Design review of the part built by this model. Coordinates are the model's own, in mm. Give positions to 0.01 mm unless a question says otherwise; leave off trailing zeros. Order: outer loops, then holes, each group sorted by start corner. A loop starts at its lowest first (then second) coordinate and runs counter-clockwise, first axis right, second up. Notation, with made-up numbers: (80.25, 29) -> (138.25, 29) arc R7 cw to (138.25, 42) -> close; hole circle Ø6 at (46.5, 56.5). An arc over 180 degrees is marked (long way). Return JSON: item names as keys, results as strings.
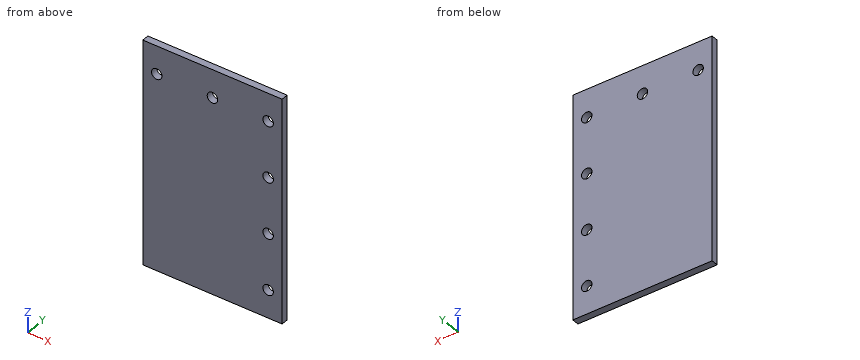
```python
from build123d import *

# Parameters (mm, degrees)
SKETCH1_W           = 63.5
SKETCH1_H           = 101.6
BOSS_EXTRUDE1_DEPTH = 3.175
SKETCH2_R           = 2.38125
CUT_EXTRUDE1_DEPTH  = 3.175


with BuildPart() as part:
    # Sketch1 → Boss-Extrude1 (new body)
    with BuildSketch(Plane(origin=(0, 0, 0), x_dir=(1, 0, 0), z_dir=(0, 1, 0))):
        Rectangle(SKETCH1_W, SKETCH1_H)
    extrude(amount=BOSS_EXTRUDE1_DEPTH)

    # Sketch2 → Cut-Extrude1 (cut)
    with BuildSketch(Plane(origin=(0, 3.175, 0), x_dir=(1, 0, 0), z_dir=(0, 1, 0))):
        with Locations(Location((25.4, -38.1, 0), (0, 0, 270))):
            Circle(SKETCH2_R)
        with Locations(Location((25.4, -12.7, 0), (0, 0, 270))):
            Circle(SKETCH2_R)
        with Locations(Location((25.4, 12.7, 0), (0, 0, 270))):
            Circle(SKETCH2_R)
        with Locations(Location((25.4, 38.1, 0), (0, 0, 270))):
            Circle(SKETCH2_R)
        with Locations(Location((0, -38.1, 0), (0, 0, 270))):
            Circle(SKETCH2_R)
        with Locations(Location((-25.4, -38.1, 0), (0, 0, 270))):
            Circle(SKETCH2_R)
        with Locations((-50.8, -38.1)):
            Circle(SKETCH2_R)
    extrude(amount=-CUT_EXTRUDE1_DEPTH, mode=Mode.SUBTRACT)


solid = part.part
```
Item 1: For pin 1 (3 mm diameter, centred on x = 25.4, z = 38.1, fed in from +Y), flat-tipped, find the tip position at first contact; note if it passes through.
Result set:
{"pin 1": "passes through"}
Item 2: Add section D-D (z = 12.7). Give the boundary of the cut face in (x, y) (3 decimals), plus the area to 3 significant figures.
Result set:
{"outline": "(-31.75, 0) -> (23.019, 0) -> (23.019, 3.175) -> (-31.75, 3.175) -> close; (27.781, 0) -> (31.75, 0) -> (31.75, 3.175) -> (27.781, 3.175) -> close", "area": "186 mm^2"}
Item 3: Add section A-A (x = 25.4). Give the boundary of the cut face in (y, z) (3 decimals), plus the area to 3 significant figures.
Result set:
{"outline": "(0, -50.8) -> (3.175, -50.8) -> (3.175, -40.481) -> (0, -40.481) -> close; (0, -35.719) -> (3.175, -35.719) -> (3.175, -15.081) -> (0, -15.081) -> close; (0, -10.319) -> (3.175, -10.319) -> (3.175, 10.319) -> (0, 10.319) -> close; (0, 15.081) -> (3.175, 15.081) -> (3.175, 35.719) -> (0, 35.719) -> close; (0, 40.481) -> (3.175, 40.481) -> (3.175, 50.8) -> (0, 50.8) -> close", "area": "262 mm^2"}
Item 4: Add section C-C (x = 0). Give the boundary of the cut face in (y, z) (3 decimals).
Result set:
{"outline": "(0, -50.8) -> (3.175, -50.8) -> (3.175, 35.719) -> (0, 35.719) -> close; (0, 40.481) -> (3.175, 40.481) -> (3.175, 50.8) -> (0, 50.8) -> close"}
Item 5: Wall thickness on L1, parallel to X at y = 0.65, z = 38.1; L2, parallel to X at y = 1.2, z = 13; L3, parallel to X at y = 2.65, z = -11: over which ranges is each line inside the solid? List them lowest first. Write a range as [from, to].
Result set:
{"L1": "x = [-31.75, -27.78], [-23.02, -2.38], [2.38, 23.02], [27.78, 31.75]", "L2": "x = [-31.75, 23.04], [27.76, 31.75]", "L3": "x = [-31.75, 23.73], [27.07, 31.75]"}
Item 6: Add section B-B (y = 2.35). Give the boundary of the cut face in (x, z).
Result set:
{"outline": "(-31.75, -50.8) -> (31.75, -50.8) -> (31.75, 50.8) -> (-31.75, 50.8) -> close; hole circle Ø4.76 at (-25.4, 38.1); hole circle Ø4.76 at (0, 38.1); hole circle Ø4.76 at (25.4, -38.1); hole circle Ø4.76 at (25.4, -12.7); hole circle Ø4.76 at (25.4, 12.7); hole circle Ø4.76 at (25.4, 38.1)"}
